Drawing for the job (mm, zero at the part's lowest x, y, z). A direction names the side the tool comes from. Round coordinates to 2 decimals unless told otherwise and drop trailing zeros. Loops run counter-clockwise (first coordinate to the right, second up) from the corner with the lowest first, then second, coordinate; pieces in that order, holes last. Notation, with made-up numbers: M -35,61 L 19,61 A27 ccw 19,85 Z; hole C 32,-33.5 d1. An arc over 180 degrees is marked long. Answer in a Markdown table with one row per item.
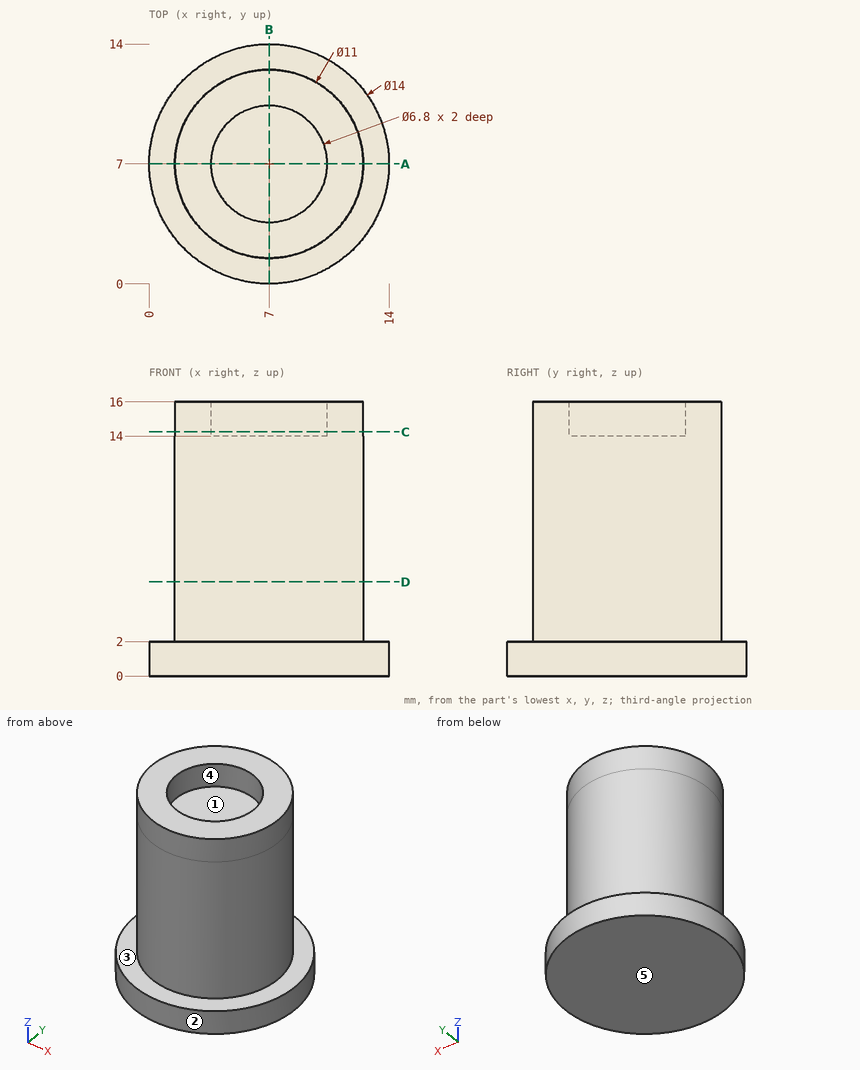
1. Mould opens along X. For the marked faces 1, 2 and 3 say: +X half, -X half, draft (parallel to the pull), parting line (faces both ways), or undercut.
Verdict:
| item | result |
|---|---|
| face 1 | undercut |
| face 2 | parting line |
| face 3 | draft |
2. Pin check, flat tips, straight feed: pin 1 (5 mm diameter, centred on x = 11, z = 10, fed in from +Y); pin 2 (4 mm diameter, centred on x = 8, y = 7, fed in from +Z); pin 3 (1 mm diameter, centred on x = 12, z = 12.5, fed in from +Y). Stop position of each tip, or through.
Verdict:
| item | result |
|---|---|
| pin 1 | stops at y = 12.29 |
| pin 2 | stops at z = 14 |
| pin 3 | stops at y = 10.16 |
3. Saw through at C-C (z = 14.25). Write the cut outline in (x, y), and give its area (3 significant figures).
Verdict:
| item | result |
|---|---|
| outline | C 7,7 d11; hole C 7,7 d6.8 |
| area | 58.7 mm² |
4. Saw through at A-A (y = 7). Write the cut outline in (x, z), and give its area (3 significant figures).
Verdict:
| item | result |
|---|---|
| outline | M 0,0 L 14,0 L 14,2 L 12.5,2 L 12.5,16 L 10.4,16 L 10.4,14 L 3.6,14 L 3.6,16 L 1.5,16 L 1.5,2 L 0,2 Z |
| area | 168 mm² |
5. Wall check: probe 1 along Z at (x, y) = (13.25, 5.25); probe 2 along Z at (x, y) = (7.75, 6.25); probe 3 along Y at (x, z) = (7, 15.3). Give the ranges that are in metal, low to high.
Verdict:
| item | result |
|---|---|
| probe 1 | z = 0 to 2 |
| probe 2 | z = 0 to 14 |
| probe 3 | y = 1.5 to 3.6, 10.4 to 12.5 |
6. Tool access for the marked faces 4 and 5: list every direction of +Z, -Z, +X, -X, +Y, -Y with a clear straight run to the whole face (end or side of a thin tool).
Verdict:
| item | result |
|---|---|
| face 4 | +Z |
| face 5 | -Z, +X, -X, +Y, -Y |
7. Saw through at D-D (z = 5.5). Write the cut outline in (x, y).
Verdict:
| item | result |
|---|---|
| outline | C 7,7 d11 |
